Source: three-view drawing plus pictorial views. Frame: mm from the lowest corner of the part. Give positions to 0.01 mm unless a question says otherwise; leave off trailing zeros. Loops run counter-clockwise (first coordinate to the right, second up) from the corner with the lowest first, then second, coordinate; pieces in that order, holes last. Notation, with made-up numbers: (49.25, 49) - (80.25, 49) arc R21 ccw to (80.25, 77) - close; hole circle Ø7 at (85, 86). An arc over 180 degrees is marked (long way). Answer as a JSON object with one key per item and string values. Group by question number.
(1) Section query D-D (x = 17.5). Return loops of the section in (y, z), plus the area to 3 significant figures.
(2) Section query B-B (y = 64). Return loops of the section in (x, z).
(3) Pin query (flat end, axial travel): P1, Ø1, axis at x = 4, z = 1, coming from the -Y side. Return the tip coordinate at first contact, or that it passes through.
(4) Material intervals for L1, parallel to Y at x = 17.5, z = 1.7; L2, parallel to X at y = 17.5, z = 1.4; L3, parallel to X at y = 64, z = 1.4, sorted ascending.
(5) Section query C-C (x = 10). Return loops of the section in (y, z), plus the area to 3 significant figures.
(6) Section query A-A (z = 1.65). Return loops of the section in (x, y).
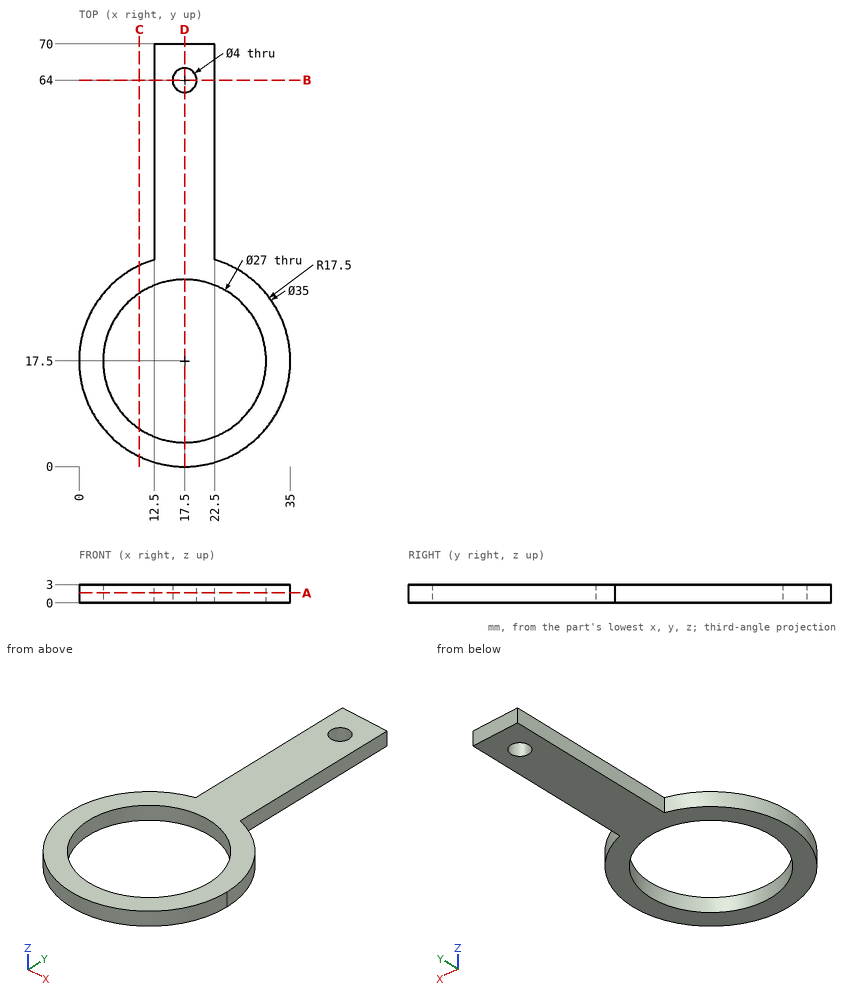
Recorded:
{
 "1": {"outline": "(0, 0) - (4, 0) - (4, 3) - (0, 3) - close; (31, 0) - (62, 0) - (62, 3) - (31, 3) - close; (66, 0) - (70, 0) - (70, 3) - (66, 3) - close", "area": "117 mm^2"},
 "2": {"outline": "(12.5, 0) - (15.5, 0) - (15.5, 3) - (12.5, 3) - close; (19.5, 0) - (22.5, 0) - (22.5, 3) - (19.5, 3) - close"},
 "3": {"P1": "stops at y = 5.78"},
 "4": {"L1": "y = 0 to 4, 31 to 62, 66 to 70", "L2": "x = 0 to 4, 31 to 35", "L3": "x = 12.5 to 15.5, 19.5 to 22.5"},
 "5": {"outline": "(1.69, 0) - (6.28, 0) - (6.28, 3) - (1.69, 3) - close; (28.72, 0) - (33.31, 0) - (33.31, 3) - (28.72, 3) - close", "area": "27.5 mm^2"},
 "6": {"outline": "(12.5, 34.27) arc R17.5 ccw (long way) to (35, 17.5) arc R17.5 ccw to (22.5, 34.27) - (22.5, 70) - (12.5, 70) - close; hole circle Ø27 at (17.5, 17.5); hole circle Ø4 at (17.5, 64)"}
}
